Geometry: see drawing. Coordinates: mm, zero at the bounding-box minimum. A direction names the side the tool comes from. Coordinates: 2 decimals unless noted, no trailing zeros. Write each loop counter-clockwise with the first axis right and the second up, starting at its lowest first coordinate (ties: lowest second). Pieces come first, ordered by that corner, then holes. Notation, with made-up numbers: (-17, 16.5) -> (7, 16.5) arc R19 ccw to (7, 42.5) -> close; hole circle Ø2 at (7.25, 68). An arc over 180 degrees is marked (long way). Use one line per item in the form item = value. Start each with the question number.
(1) Cut plane B-B on z = 7.75. Return the cut outline in (x, y), plus the area to 4 significant figures.
(2) Set-up query: the marked faces 4 and 5. Return all of +Z, -Z, +X, -X, +Y, -Y with unobstructed straight access to the full face (end or side cutting, diameter ignored); none if empty.
(3) Cut plane A-A on x = 7.75. Return the cut outline in (y, z), plus the area to 4 significant figures.
(4) Cut plane C-C on y = 4. Return the cut outline in (x, z), plus the area to 3 significant figures.
(5) Pull-direction query (Z, two-part tool) for the marked faces 1, 2 and 3; classes: released by +Z, released by -Z, zero draft, split by the parting line, or undercut.
(6) First-contact query: pin 1 (5 mm diameter, centred on y = 6, z = 12.5, fed in from +X); pin 2 (3.5 mm diameter, centred on x = 7.75, z = 7.75, fed in from -Y); pin 3 (1 mm diameter, centred on x = 11, z = 2, fed in from +Y). Flat tips, straight axial feed; report the tip coordinate or a pass-through.
(7) Ray query, line 1 along Z through (x, y) = (7.75, 1.5); line 2 along Y through (x, z) = (10.5, 7.5); line 3 along Y through (x, z) = (7, 3.5). Return the intervals inside material, ascending.
(8) Cut plane D-D on z = 5. Return the cut outline in (x, y).
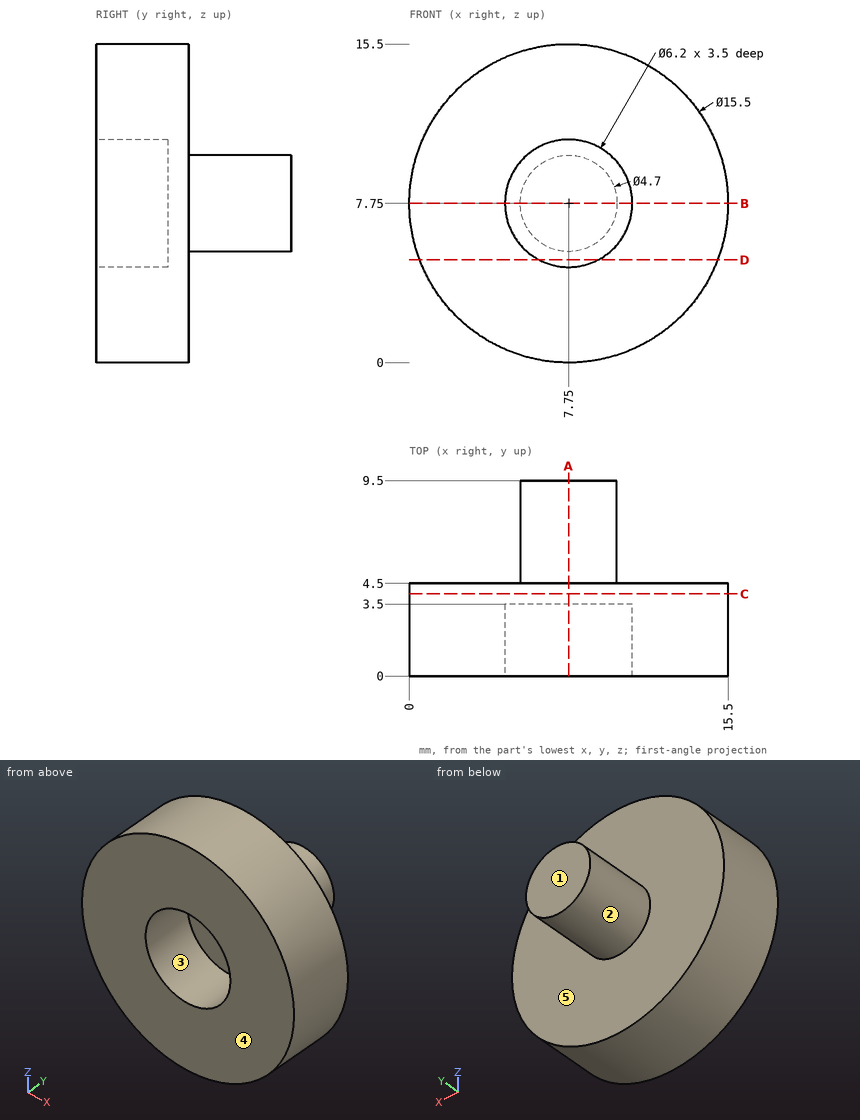
Values:
q1.outline = (0, 0) -> (4.65, 0) -> (4.65, 3.5) -> (10.85, 3.5) -> (10.85, 0) -> (15.5, 0) -> (15.5, 4.5) -> (10.1, 4.5) -> (10.1, 9.5) -> (5.4, 9.5) -> (5.4, 4.5) -> (0, 4.5) -> close
q1.area = 71.55 mm2
q2.face_4 = +Z, -Z, +X, -X, -Y
q2.face_5 = +Y
q3.outline = (0, 0) -> (4.5, 0) -> (4.5, 5.4) -> (9.5, 5.4) -> (9.5, 10.1) -> (4.5, 10.1) -> (4.5, 15.5) -> (0, 15.5) -> (0, 10.85) -> (3.5, 10.85) -> (3.5, 4.65) -> (0, 4.65) -> close
q3.area = 71.55 mm2
q4.outline = circle Ø15.5 at (7.75, 7.75)
q4.area = 189 mm2
q5.face_1 = zero draft
q5.face_2 = split by the parting line
q5.face_3 = undercut
q6.pin_1 = 15
q6.pin_2 = 3.5
q6.pin_3 = 4.5
q7.line_1 = 0 to 4.65, 10.85 to 15.5
q7.line_2 = 3.5 to 4.5
q7.line_3 = 0 to 4.5
q8.outline = (0.5, 0) -> (6.32, 0) -> (6.32, 3.5) -> (9.18, 3.5) -> (9.18, 0) -> (15, 0) -> (15, 4.5) -> (0.5, 4.5) -> close
